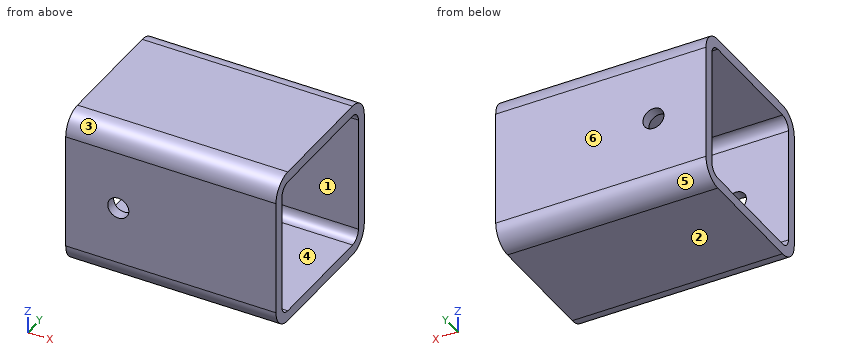
```python
from build123d import *

# Parameters (mm, degrees)
EXTRUDE_1_DEPTH          = 20
CUT_EXTRUDE_1_DEPTH      = 30.154759474
CUT_EXTRUDE_1_DEPTH_BACK = 30.154759474
SKETCH_2_R               = 2


with BuildPart() as part:
    # 草图1 → 凸台-拉伸1 (new, symmetric)
    with BuildSketch(Plane(origin=(0, 0, 0), x_dir=(0, 0, -1), z_dir=(1, 0, 0))):
        with BuildLine():
            Line((-11, -15), (11, -15))
            ThreePointArc((11, -15), (13.828427125, -13.828427125), (15, -11))
            Line((15, -11), (15, 11))
            ThreePointArc((15, 11), (13.828427125, 13.828427125), (11, 15))
            Line((11, 15), (-11, 15))
            ThreePointArc((-11, 15), (-13.828427125, 13.828427125), (-15, 11))
            Line((-15, 11), (-15, -11))
            ThreePointArc((-15, -11), (-13.828427125, -13.828427125), (-11, -15))
        make_face()
        with BuildLine():
            Line((-11, -13), (11, -13))
            ThreePointArc((11, -13), (12.414213562, -12.414213562), (13, -11))
            Line((13, -11), (13, 11))
            ThreePointArc((13, 11), (12.414213562, 12.414213562), (11, 13))
            Line((11, 13), (-11, 13))
            ThreePointArc((-11, 13), (-12.414213562, 12.414213562), (-13, 11))
            Line((-13, 11), (-13, -11))
            ThreePointArc((-13, -11), (-12.414213562, -12.414213562), (-11, -13))
        make_face(mode=Mode.SUBTRACT)
    extrude(amount=EXTRUDE_1_DEPTH, both=True)

    # 草图2 → 切除-拉伸1 (cut, two sides: drawn at the far end of the back side and taken through both)
    with BuildSketch(Plane(origin=(0, 0, 0), x_dir=(1, 0, 0), z_dir=(0, 1, 0)).offset(-CUT_EXTRUDE_1_DEPTH_BACK)):
        with Locations(Location((-10, 0, 0), (0, 0, 270))):
            Circle(SKETCH_2_R)
    extrude(amount=CUT_EXTRUDE_1_DEPTH + CUT_EXTRUDE_1_DEPTH_BACK, mode=Mode.SUBTRACT)


solid = part.part
```
Model file for the job. Use its own axes, mm. Face numbers are marked on the shaded views. A direction names the side the tool comes from. Coordinates: 2 decimals unless noted, no trailing zeros. Loops run counter-clockwise (first coordinate to the right, second up) from the corner with the lowest first, then second, coordinate; pieces in that order, holes last. Notation, with made-up numbers: (56.25, 9.25) - (95.25, 9.25) arc R31 ccw to (95.25, 44.25) - close; hole circle Ø4 at (25, 2). An arc over 180 degrees is marked (long way). Answer as a JSON object with one key per item and string values. Group by question number.
(1) Cut at C-C (x = 7.5). Give the cut face in (y, z), then the cut area to 3 significant figures.
(2) Cut at D-D (z = 0.5). Give the cut face in (x, y).
(3) Two-plate mould, pull along Z, no slides. Class the marked faces 3, 4, 5 and 6: released by +Z, released by -Z, zero draft, split by the parting line, or undercut.
(4) Tool access for the marked faces 1 and 2: list every direction of +Z, -Z, +X, -X, +Y, -Y with a clear straight run to the whole face (end or side of a thin tool).
(5) Cut at A-A (z = -2.75). Give the cut face in (x, y), then the cut area to 3 significant figures.
(6) Probe line 1 along Z through (x, y) = (12, -8); line 2 along X through (y, z) = (14.45, 0). List the from-to ranges inside material, lowest first.
Geometry says:
{
 "1": {"outline": "(-15, -11) arc R4 ccw to (-11, -15) - (11, -15) arc R4 ccw to (15, -11) - (15, 11) arc R4 ccw to (11, 15) - (-11, 15) arc R4 ccw to (-15, 11) - close; hole (-13, -11) arc R2 ccw to (-11, -13) - (11, -13) arc R2 ccw to (13, -11) - (13, 11) arc R2 ccw to (11, 13) - (-11, 13) arc R2 ccw to (-13, 11) - close", "area": "214 mm^2"},
 "2": {"outline": "(-20, -15) - (-11.94, -15) - (-11.94, -13) - (-20, -13) - close; (-20, 13) - (-11.94, 13) - (-11.94, 15) - (-20, 15) - close; (-8.06, -15) - (20, -15) - (20, -13) - (-8.06, -13) - close; (-8.06, 13) - (20, 13) - (20, 15) - (-8.06, 15) - close"},
 "3": {"face 3": "released by +Z", "face 4": "undercut", "face 5": "released by -Z", "face 6": "zero draft"},
 "4": {"face 1": "+X, -X", "face 2": "-Z, +X, -X, +Y, -Y"},
 "5": {"outline": "(-20, -15) - (20, -15) - (20, -13) - (-20, -13) - close; (-20, 13) - (20, 13) - (20, 15) - (-20, 15) - close", "area": "160 mm^2"},
 "6": {"line 1": "z = -15 to -13, 13 to 15", "line 2": "x = -20 to -12, -8 to 20"}
}
